Source: CAD feature listing. Evaluate the final solid. Frame: model axes, mm. A direction names the side the tool comes from. Give positions to 0.01 mm unless a question says otherwise; leave off trailing zeros. Write each loop counter-clockwise with the first axis right and the second up, starting at its lowest first coordinate (ties: lowest second). Pieces come first, ordered by that corner, then holes. Notation, with made-up numbers: (-37.5, 82) -> (-3.5, 82) arc R9 cw to (-3.5, 99) -> close; hole circle Ø11 at (-24.75, 59). An arc over 180 degrees is marked (long way). Answer as a JSON object with one key per item and string values. Group by question number.
Item 1: Section query A-A on y = 2.65. Return the cut outline in (x, z).
Item 2: Section query D-D on x = 12.5. Return the cut outline in (y, z), plus the area to 3 significant figures.
Item 3: Section query C-C on z = -13.75. Return the cut outline in (x, y), plus the area to 3 significant figures.
Item 4: Section query B-B on x = 18.5. Return the cut outline in (y, z).
Item 5: Ray query, probe 1 along X at (y, z) = (1.15, -10); probe 2 along X at (y, z) = (1.35, -9.5); probe 3 along Y at (x, z) = (5.75, -6.5). Return the intervals inside material, ascending. Write a range as from..to.
Item 6: Pull-direction query (Z, two-part tool) for faces 1 (the face through (0, 1, -10)), 2 (the face through (2, 2, -17.19)), 3 (the face through (1.01, 0.86, -10.63)), 4 (the face through (10, 1, 0)); classes: pulls with the +Z half, pulls with the -Z half, needs draft (parallel to the pull), parting line crosses it, or undercut.
Item 7: First-contact query: pin 1 Ø1.3 at (x, z) = (1.5, -10) entering from +Y; pin 2 Ø0.6 at (x, z) = (10, -3) entering from -Y. Flat tips, straight axial feed; report the tip coordinate or a pass-through.
Item 8: Access query for faces 5 (the face through (4, 2, -1.558)), 6 (the face through (4, 2, -4.684)), 7 (the face through (6.973, 2, -3)), 8 (the face through (1.313, 2, -3)), 9 (the face through (1.008, 2, -15)). Directions: +Z, -Z, +X, -X, +Y, -Y. A direction counts if a zero-diameter tool reaches every point of the face in a straight line with its end or side. Return the directions, or none.
from build123d import *

# Parameters (mm, degrees)
SKETCH_1_W          = 20
SKETCH_1_H          = 20
EXTRUDE_1_DEPTH     = 1.7
SKETCH_2_W          = 0.7
SKETCH_2_H          = 1.5
CUT_EXTRUDE_1_DEPTH = 0.05
SKETCH_3_R          = 0.8
CUT_EXTRUDE_2_DEPTH = 29.335313656
SKETCH_6_W          = 5.659546013
SKETCH_6_H          = 3.125880025
EXTRUDE_4_DEPTH     = 1.3
SKETCH_7_W          = 1.909465354
SKETCH_7_H          = 3.796411433
EXTRUDE_5_DEPTH     = 1.4


with BuildPart() as part:
    # 스케치1 → 보스-돌출1 (new body)
    with BuildSketch(Plane(origin=(0, 0, 0), x_dir=(1, 0, 0), z_dir=(0, 1, 0))):
        with Locations((10, 10)):
            Rectangle(SKETCH_1_W, SKETCH_1_H)
    extrude(amount=EXTRUDE_1_DEPTH)

    # 스케치2 → 컷-돌출1 (cut)
    with BuildSketch(Plane(origin=(0, 0, 0), x_dir=(1, 0, 0), z_dir=(0, 1, 0))):
        with Locations((2.38, 2.75)):
            Rectangle(SKETCH_2_W, SKETCH_2_H)
        with Locations((3.65, 2.75)):
            Rectangle(SKETCH_2_W, SKETCH_2_H)
        with Locations((4.92, 2.75)):
            Rectangle(SKETCH_2_W, SKETCH_2_H)
        with Locations((6.19, 2.75)):
            Rectangle(SKETCH_2_W, SKETCH_2_H)
        with Locations((7.46, 2.75)):
            Rectangle(SKETCH_2_W, SKETCH_2_H)
        with Locations((8.73, 2.75)):
            Rectangle(SKETCH_2_W, SKETCH_2_H)
        with Locations((10, 2.75)):
            Rectangle(SKETCH_2_W, SKETCH_2_H)
        with Locations((11.27, 2.75)):
            Rectangle(SKETCH_2_W, SKETCH_2_H)
        with Locations((12.54, 2.75)):
            Rectangle(SKETCH_2_W, SKETCH_2_H)
        with Locations((13.81, 2.75)):
            Rectangle(SKETCH_2_W, SKETCH_2_H)
        with Locations((15.08, 2.75)):
            Rectangle(SKETCH_2_W, SKETCH_2_H)
        with Locations((16.35, 2.75)):
            Rectangle(SKETCH_2_W, SKETCH_2_H)
        with Locations((17.62, 2.75)):
            Rectangle(SKETCH_2_W, SKETCH_2_H)
    extrude(amount=CUT_EXTRUDE_1_DEPTH, mode=Mode.SUBTRACT)

    # 스케치3 → 컷-돌출2 (cut, through all)
    with BuildSketch(Plane(origin=(0, 1.7, 0), x_dir=(1, 0, 0), z_dir=(0, 1, 0))):
        with Locations(Location((1.5, 10, 0), (0, 0, 270))):
            Circle(SKETCH_3_R)
        with Locations(Location((18.5, 10, 0), (0, 0, 270))):
            Circle(SKETCH_3_R)
    extrude(amount=-CUT_EXTRUDE_2_DEPTH, mode=Mode.SUBTRACT)

    # 스케치6 → 보스-돌출4 (add)
    with BuildSketch(Plane(origin=(0, 1.7, 0), x_dir=(1, 0, 0), z_dir=(0, 1, 0))):
        with Locations((4.142822267, 3.120933029)):
            Rectangle(SKETCH_6_W, SKETCH_6_H)
    extrude(amount=EXTRUDE_4_DEPTH)

    # 스케치7 → 보스-돌출5 (add)
    with BuildSketch(Plane(origin=(0, 1.7, 0), x_dir=(1, 0, 0), z_dir=(0, 1, 0))):
        with Locations((1.96252084, 15.291638164)):
            Rectangle(SKETCH_7_W, SKETCH_7_H)
    extrude(amount=EXTRUDE_5_DEPTH)


solid = part.part
Worked answers:
{
 "1": {"outline": "(1.01, -17.19) -> (2.92, -17.19) -> (2.92, -13.39) -> (1.01, -13.39) -> close; (1.31, -4.68) -> (6.97, -4.68) -> (6.97, -1.56) -> (1.31, -1.56) -> close"},
 "2": {"outline": "(0, -20) -> (1.7, -20) -> (1.7, 0) -> (0, 0) -> (0, -2) -> (0.05, -2) -> (0.05, -3.5) -> (0, -3.5) -> close", "area": "33.9 mm^2"},
 "3": {"outline": "(0, 0) -> (20, 0) -> (20, 1.7) -> (2.92, 1.7) -> (2.92, 3.1) -> (1.01, 3.1) -> (1.01, 1.7) -> (0, 1.7) -> close", "area": "36.7 mm^2"},
 "4": {"outline": "(0, -20) -> (1.7, -20) -> (1.7, -10.8) -> (0, -10.8) -> close; (0, -9.2) -> (1.7, -9.2) -> (1.7, 0) -> (0, 0) -> close"},
 "5": {"probe 1": "0..0.7, 2.3..17.7, 19.3..20", "probe 2": "0..0.88, 2.12..17.88, 19.12..20", "probe 3": "0..1.7"},
 "6": {"face 1": "needs draft", "face 2": "pulls with the -Z half", "face 3": "undercut", "face 4": "pulls with the +Z half"},
 "7": {"pin 1": "through", "pin 2": "y = 0.05"},
 "8": {"face 5": "+Z, +X, -X, +Y", "face 6": "+X, -X, +Y", "face 7": "+Z, -Z, +X, +Y", "face 8": "+Z, -X, +Y", "face 9": "+Z, -Z, -X, +Y"}
}
